```python
from build123d import *

# Parameters (mm, degrees)
F0_R        = 9.8
F0_R_2      = 6.1
F0_R_3      = 4.6
F1_DEPTH    = 2
F2_R        = 2
F3_R        = 3
F4_W        = 40
F4_H        = 8
F5_DEPTH    = 25
F6_R        = 2
F7_R        = 8
F8_R        = 12
F9_C1_SIZE2 = 4.5
F9_C1_SIZE  = 9.5
F9_C2_SIZE2 = 9.5
F9_C2_SIZE  = 4.5
F9_C3_SIZE2 = 9.5
F9_C3_SIZE  = 4.5
F9_C4_SIZE2 = 9.5
F9_C4_SIZE  = 4.5


# Not quite as in the source:
# - two fillets or chamfers of one size are made in one step


with BuildPart() as f1:
    # F0 (on Top) → F1 (new body)
    with BuildSketch(Plane.XY):
        with BuildLine():
            Line((36, 40.6180607378), (-36, 40.6180607378))
            Line((-36, 40.6180607378), (-36, 78.6180607378))
            Line((-36, 78.6180607378), (-59, 78.6180607378))
            Line((-59, 78.6180607378), (-59, 40.6180607378))
            Line((-59, 40.6180607378), (-59, 34.2180607378))
            Line((-59, 34.2180607378), (-52.466149277, 15.0342559872))
            Line((-52.466149277, 15.0342559872), (-49.3893506198, 6.000577809))
            Line((-49.3893506198, 6.000577809), (-63.7943902368, 1.0943363339))
            ThreePointArc((-63.7943902368, 1.0943363339), (-72.5331453979, -16.6717594171), (-54.7670496468, -25.4105145782))
            Line((-54.7670496468, -25.4105145782), (-40.3620100298, -20.5042731031))
            Line((-40.3620100298, -20.5042731031), (-34.2730196821, -38.3819392622))
            Line((-34.2730196821, -38.3819392622), (34.5899127424, -38.3819392622))
            Line((34.5899127424, -38.3819392622), (59, 34.2180607378))
            Line((59, 34.2180607378), (59, 40.6180607378))
            Line((59, 40.6180607378), (59, 78.6180607378))
            Line((59, 78.6180607378), (36, 78.6180607378))
            Line((36, 78.6180607378), (36, 40.6180607378))
        make_face()
        with Locations((-59.2807199418, -12.1580891221)):
            Circle(F0_R, mode=Mode.SUBTRACT)
        with Locations((-25.5, -27.7819392622)):
            Circle(F0_R_2, mode=Mode.SUBTRACT)
        with Locations((25.5, -27.7819392622)):
            Circle(F0_R_2, mode=Mode.SUBTRACT)
        with BuildLine():
            ThreePointArc((-28, 2.2180607378), (-27.4142135624, 3.6322743002), (-26, 4.2180607378))
            Line((-26, 4.2180607378), (25, 4.2180607378))
            ThreePointArc((25, 4.2180607378), (27.1213203436, 3.3393810814), (28, 1.2180607378))
            Line((28, 1.2180607378), (28, -16.7819392622))
            ThreePointArc((28, -16.7819392622), (27.1213203436, -18.9032596057), (25, -19.7819392622))
            Line((25, -19.7819392622), (19.5, -19.7819392622))
            ThreePointArc((19.5, -19.7819392622), (17.3786796564, -20.6606189186), (16.5, -22.7819392622))
            Line((16.5, -22.7819392622), (16.5, -24.0702618733))
            ThreePointArc((16.5, -24.0702618733), (15.6213203436, -26.1915822169), (13.5, -27.0702618733))
            Line((13.5, -27.0702618733), (-13.5, -27.0702618733))
            ThreePointArc((-13.5, -27.0702618733), (-15.6213203436, -26.1915822169), (-16.5, -24.0702618733))
            Line((-16.5, -24.0702618733), (-16.5, -22.7819392622))
            ThreePointArc((-16.5, -22.7819392622), (-17.3786796564, -20.6606189186), (-19.5, -19.7819392622))
            Line((-19.5, -19.7819392622), (-25, -19.7819392622))
            ThreePointArc((-25, -19.7819392622), (-27.1213203436, -18.9032596057), (-28, -16.7819392622))
            Line((-28, -16.7819392622), (-28, 2.2180607378))
        make_face(mode=Mode.SUBTRACT)
        with Locations((-47.5, 34.2180607378)):
            Circle(F0_R_3, mode=Mode.SUBTRACT)
        with Locations((-47.5, 69.2180607378)):
            Circle(F0_R_3, mode=Mode.SUBTRACT)
        Polygon((-20, 18.6180607378), (-34, 18.6180607378), (-34, 23.6180607378), (-20, 23.6180607378), (-20, 26.1180607378), (20, 26.1180607378), (20, 23.6180607378), (34, 23.6180607378), (34, 18.6180607378), (20, 18.6180607378), (20, 16.1180607378), (-20, 16.1180607378), align=None, mode=Mode.SUBTRACT)
        with Locations((47.5, 34.2180607378)):
            Circle(F0_R_3, mode=Mode.SUBTRACT)
        with Locations((47.5, 69.2180607378)):
            Circle(F0_R_3, mode=Mode.SUBTRACT)
    extrude(amount=F1_DEPTH)

    # F2
    f2_edges = [f1.edges().sort_by_distance(p)[0] for p in [
        (59, 34.218061, 1),
        (-20, 26.118061, 1),
        (20, 23.618061, 1),
        (-34, 23.618061, 1),
        (-20, 18.618061, 1),
        (-34, 18.618061, 1),
        (20, 18.618061, 1),
        (34, 23.618061, 1),
        (34, 18.618061, 1),
        (-59, 34.218061, 1),
        (-36, 40.618061, 1),
        (36, 40.618061, 1),
    ]]
    fillet(f2_edges, radius=F2_R)

    # F3
    f3_edges = [f1.edges().sort_by_distance(p)[0] for p in [
        (-20, 23.618061, 1),
        (-20, 16.118061, 1),
        (20, 26.118061, 1),
        (20, 16.118061, 1),
        (-34.27302, -38.381939, 1),
        (34.589913, -38.381939, 1),
    ]]
    fillet(f3_edges, radius=F3_R)

    # F4 (on face) → F5 (cut)
    with BuildSketch(Plane.XY.offset(2)):
        with Locations((0.2679491924, 36.6180607378)):
            Rectangle(F4_W, F4_H)
    extrude(amount=-F5_DEPTH, mode=Mode.SUBTRACT)

    # F6
    f6_edges = [f1.edges().sort_by_distance(p)[0] for p in [
        (-19.732051, 40.618061, 1),
        (-19.732051, 32.618061, 1),
        (20.267949, 40.618061, 1),
        (20.267949, 32.618061, 1),
    ]]
    fillet(f6_edges, radius=F6_R)

    # F7
    f7_edges = [f1.edges().sort_by_distance(p)[0] for p in [
        (-40.36201, -20.504273, 1),
    ]]
    fillet(f7_edges, radius=F7_R)

    # F8
    f8_edges = [f1.edges().sort_by_distance(p)[0] for p in [
        (-49.389351, 6.000578, 1),
    ]]
    fillet(f8_edges, radius=F8_R)

    # F9: chamfer of 9.5 x 4.5 on 4 edges, made by hand

    # F9_c1
    f9_c1_edges = [f1.edges().sort_by_distance(p)[0] for p in [
        (-59, 78.6180607378, 1),
    ]]
    f9_c1_side = f1.faces().sort_by_distance((-59, 78.5280607378, 1))[0]
    chamfer(f9_c1_edges, length=F9_C1_SIZE, length2=F9_C1_SIZE2, reference=f9_c1_side)

    # F9_c2
    f9_c2_edges = [f1.edges().sort_by_distance(p)[0] for p in [
        (-36, 78.6180607378, 1),
    ]]
    f9_c2_side = f1.faces().sort_by_distance((-36.09, 78.6180607378, 1))[0]
    chamfer(f9_c2_edges, length=F9_C2_SIZE, length2=F9_C2_SIZE2, reference=f9_c2_side)

    # F9_c3
    f9_c3_edges = [f1.edges().sort_by_distance(p)[0] for p in [
        (59, 78.6180607378, 1),
    ]]
    f9_c3_side = f1.faces().sort_by_distance((58.91, 78.6180607378, 1))[0]
    chamfer(f9_c3_edges, length=F9_C3_SIZE, length2=F9_C3_SIZE2, reference=f9_c3_side)

    # F9_c4
    f9_c4_edges = [f1.edges().sort_by_distance(p)[0] for p in [
        (36, 78.6180607378, 1),
    ]]
    f9_c4_side = f1.faces().sort_by_distance((36.09, 78.6180607378, 1))[0]
    chamfer(f9_c4_edges, length=F9_C4_SIZE, length2=F9_C4_SIZE2, reference=f9_c4_side)


solid = f1.part
```
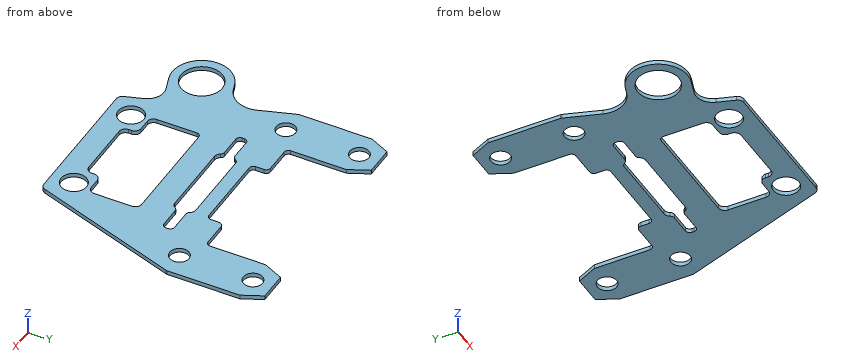
The model under review builds one solid part; all positions refer to its coordinate system, in mm. Give positions to 0.01 mm unless a question says otherwise; leave off trailing zeros. Order: outer loops, then holes, each group sorted by start corner. A loop starts at its lowest first (then second) coordinate and runs counter-clockwise, first axis right, second up. Notation, with made-up numbers: (-18.5, 83) - (35.5, 83) arc R19 cw to (35.5, 116) - close; hole circle Ø8 at (-28, 38). An arc over 180 degrees is marked (long way). Use CSV: the item, a comma, the result in double quotes. Start each with the question number.
Q1. We need section D-D, the plane z = 1.15. State how many separate pieces and enclosed holes the cut face has, and give its area (3 significant figures).
Q2. We need section B-B, the plane x = -12. Write out the cut boundary in (y, z), and give its area (3 significant figures).
Q3. Clearance check with flat-ended pins moving along their axes: pin 1 Ø1 at (y, z) = (5.5, 1) entering from +X; pin 2 Ø0.6 at (x, z) = (-4, 1.5) entering from +Y; pin 3 Ø0.6 at (y, z) = (-11.5, 1) entering from +X. State where each tip first meets the part, or that it passes through.
Q4. We need section A-A, the plane y = 45. Write out the cut boundary in (x, z).
Q5. We need section C-C, the plane x = 47.5. Write out the cut boundary in (y, z), and give its area (3 significant figures).
Q6. To check wall thickness, follow line 1 along X through (y, z) = (69, 1.1); line 2 along Y through (x, z) = (-12.5, 0.65); line 3 along X through (y, z) = (36, 1.9). State the ranges of each line that lie inside material, in increasing order. Write a range as [from, to].
Outcome:
1,separate pieces,"1"
1,enclosed holes,"9"
1,area,"6,740 mm^2"
2,outline,"(-38.38, 0) - (-27.07, 0) - (-27.07, 2) - (-38.38, 2) - close; (4.22, 0) - (16.12, 0) - (16.12, 2) - (4.22, 2) - close; (26.12, 0) - (32.62, 0) - (32.62, 2) - (26.12, 2) - close"
2,area,"59.4 mm^2"
3,pin 1,"stops at x = 49.51"
3,pin 2,"stops at y = 32.62"
3,pin 3,"stops at x = 43.73"
4,outline,"(-59, 0) - (-36, 0) - (-36, 2) - (-59, 2) - close; (36, 0) - (59, 0) - (59, 2) - (36, 2) - close"
5,outline,"(0.01, 0) - (29.62, 0) - (29.62, 2) - (0.01, 2) - close; (38.82, 0) - (64.62, 0) - (64.62, 2) - (38.82, 2) - close; (73.82, 0) - (78.62, 0) - (78.62, 2) - (73.82, 2) - close"
5,area,"120 mm^2"
6,line 1,"x = [-59, -52.09], [-42.91, -36], [36, 42.91], [52.09, 59]"
6,line 2,"y = [-38.38, -27.07], [4.22, 16.12], [26.12, 32.62]"
6,line 3,"x = [-59, -51.74], [-43.26, -19.73], [20.27, 43.26], [51.74, 59]"
